For this review, take the finished solid that the model builds, in its own axes (mm). A direction names the side the tool comes from. Round coordinates to 2 decimals unless told otherwise and drop trailing zeros. Order: outer loops, then holes, each group sorted by start corner. A loop starts at its lowest first (then second) coordinate and runs counter-clockwise, first axis right, second up. Notation, with made-up numbers: (-30, 11) -> (-14, 11) arc R16 ccw to (-14, 25) -> close; hole circle Ø10 at (-29, 61). An arc over 180 degrees is marked (long way). Use a Markdown table: item, result. Add a question column.
1) Consider section C-C (x = 70). State the section outline as (y, z) points.
2) Clearance check with flat-ended pins moving along their axes: P1, Ø3, axis at x = -5.66, z = -5.66, coming from the +Y side; P2, Ø1, axis at y = 6, z = 49.5, coming from the -X side; P3, Ø6, axis at x = 40.5, y = 6.5, coming from the +Z side; P4, Ø3, axis at x = 2.5, z = 82.5, coming from the +Y side. State where each tip first meets the part, or that it passes through.
3) Consider section B-B (z = 75). State the section outline as (x, y) points, plus the area to 3 significant figures.
4) Consider section A-A (y = 6.75). State the section outline as (x, z) points, plus the area to 3 significant figures.
5) Machinability: for faces 1 (the face through (5, 5, 50)), 2 (the face through (-5, 5, -50)), 3 (the face through (50, 5, -5)), 4 (the face through (0, 7, 78.1)), 5 (the face through (78.1, 7, 0)), which of the approach directions +Z, -Z, +X, -X, +Y, -Y give a long, thin tool a straight path to every point of the face, cutting with its end or side? Answer none if there is none.
6) Wall thickness on line 1 along X through (y, z) = (3.7, 0); line 2 along Z through (x, y) = (-83.2, 3.4); line 3 along X through (y, z) = (4.5, 50): over which ranges is each line inside the solid? List them lowest first. Write a range as [from, to].
```python
from build123d import *

# Parameters (mm, degrees)
SKETCH1_R           = 11.95
BOSS_EXTRUDE1_DEPTH = 10
BOSS_EXTRUDE2_DEPTH = 10
CUT_EXTRUDE2_DEPTH  = 17.95
SKETCH6_R           = 1.75
CUT_EXTRUDE4_DEPTH  = 10
CIRPATTERN2_COUNT   = 4
SKETCH5_R           = 1.75
CUT_EXTRUDE3_DEPTH  = 11


with BuildPart() as part:
    # Sketch1 → Boss-Extrude1 (new body)
    with BuildSketch(Plane(origin=(0, 0, 0), x_dir=(1, 0, 0), z_dir=(0, 1, 0))):
        Circle(SKETCH1_R)
    extrude(amount=BOSS_EXTRUDE1_DEPTH)

    # Sketch2 → Boss-Extrude2 (add)
    with BuildSketch(Plane(origin=(0, 10, 0), x_dir=(1, 0, 0), z_dir=(0, 1, 0))):
        with BuildLine():
            Line((10.85368601, -5), (98.2, -5))
            Line((98.2, -5), (98.2, 5))
            Line((98.2, 5), (10.85368601, 5))
            ThreePointArc((10.85368601, 5), (11.95, 0), (10.85368601, -5))
        make_face()
    boss_extrude2 = extrude(amount=-BOSS_EXTRUDE2_DEPTH)

    # Sketch4 → Cut-Extrude2 (cut, through all)
    with BuildSketch(Plane.XY.offset(5)):
        Polygon((88.1, 0), (88.1, 4.9), (78.1, 4.9), (78.1, 10), (98.2, 10), (98.2, 0), align=None)
    cut_extrude2 = extrude(amount=-CUT_EXTRUDE2_DEPTH, mode=Mode.SUBTRACT)

    # Sketch6 → Cut-Extrude4 (cut)
    with BuildSketch(Plane(origin=(0, 4.9, 0), x_dir=(1, 0, 0), z_dir=(0, 1, 0))):
        with Locations((83.2, 0)):
            Circle(SKETCH6_R)
    cut_extrude4 = extrude(amount=-CUT_EXTRUDE4_DEPTH, mode=Mode.SUBTRACT)

    # CirPattern2: Boss-Extrude2, Cut-Extrude2, Cut-Extrude4 ×4 about axis
    cirpattern2_axis = Axis((0, 0, 0), (0, 1, 0))
    for i in range(1, CIRPATTERN2_COUNT):
        add(boss_extrude2.rotate(cirpattern2_axis, i * 360 / CIRPATTERN2_COUNT))
        add(cut_extrude2.rotate(cirpattern2_axis, i * 360 / CIRPATTERN2_COUNT), mode=Mode.SUBTRACT)
        add(cut_extrude4.rotate(cirpattern2_axis, i * 360 / CIRPATTERN2_COUNT), mode=Mode.SUBTRACT)

    # Sketch5 → Cut-Extrude3 (cut, through all)
    with BuildSketch(Plane(origin=(0, 10, 0), x_dir=(1, 0, 0), z_dir=(0, 1, 0))):
        with Locations((5.656854249, 5.656854249)):
            Circle(SKETCH5_R)
        with Locations((5.656854249, -5.656854249)):
            Circle(SKETCH5_R)
        with Locations((-5.656854249, -5.656854249)):
            Circle(SKETCH5_R)
        with Locations((-5.656854249, 5.656854249)):
            Circle(SKETCH5_R)
    extrude(amount=-CUT_EXTRUDE3_DEPTH, mode=Mode.SUBTRACT)


solid = part.part
```
Results list:
| question | item | result |
|---|---|---|
| 1 | outline | (0, -5) -> (10, -5) -> (10, 5) -> (0, 5) -> close |
| 2 | P1 | through |
| 2 | P2 | x = -5 |
| 2 | P3 | z = 5 |
| 2 | P4 | y = 4.9 |
| 3 | outline | (-5, 0) -> (5, 0) -> (5, 10) -> (-5, 10) -> close |
| 3 | area | 100 mm2 |
| 4 | outline | (-78.1, -5) -> (-10.85, -5) arc R11.95 ccw to (-5, -10.85) -> (-5, -78.1) -> (5, -78.1) -> (5, -10.85) arc R11.95 ccw to (10.85, -5) -> (78.1, -5) -> (78.1, 5) -> (10.85, 5) arc R11.95 ccw to (5, 10.85) -> (5, 78.1) -> (-5, 78.1) -> (-5, 10.85) arc R11.95 ccw to (-10.85, 5) -> (-78.1, 5) -> close; hole circle Ø3.5 at (-5.66, -5.66); hole circle Ø3.5 at (-5.66, 5.66); hole circle Ø3.5 at (5.66, -5.66); hole circle Ø3.5 at (5.66, 5.66) |
| 4 | area | 3,070 mm2 |
| 5 | face 1 | +Z, +X, +Y, -Y |
| 5 | face 2 | -Z, -X, +Y, -Y |
| 5 | face 3 | -Z, +X, +Y, -Y |
| 5 | face 4 | +Z, +X, -X, +Y |
| 5 | face 5 | +Z, -Z, +X, +Y |
| 6 | line 1 | [-88.1, -84.95], [-81.45, 81.45], [84.95, 88.1] |
| 6 | line 2 | [-5, -1.75], [1.75, 5] |
| 6 | line 3 | [-5, 5] |
